Autodesk Fusion 360 part; units mm, degrees
sketch "Skizze1" plane through (0, 0, 0) normal (0, 0, 1) x (1, 0, 0)
  line L0 (0, 0) -> (200, 0)
  line L1 (200, 0) -> (200, 24)
  line L2 (200, 24) -> (0, 24)
  line L3 (0, 24) -> (0, 0)
  line L4 (2, 2) -> (198, 2)
  line L5 (198, 2) -> (198, 22)
  line L6 (198, 22) -> (2, 22)
  line L7 (2, 22) -> (2, 2)
  dimension "d1" = 200
  dimension "d2" = 24
extrude "Extrusion1" add sketch "Skizze1" along normal blind 2 contours L4 L5 L6 L7
extrude "Extrusion2" add sketch "Skizze1" along normal blind 124
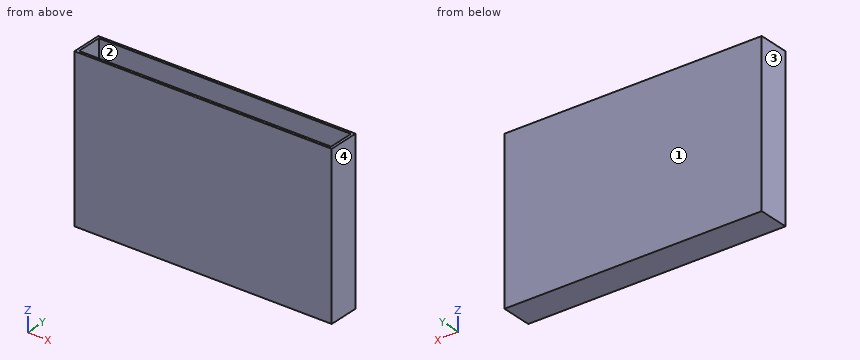
The model under review builds one solid part; all positions refer to its coordinate system, in mm. Face numbers are marked on the shaded views. Give positions to 0.01 mm unless a question says otherwise; leave off trailing zeros. Order: outer loops, then holes, each group sorted by start corner. A loop starts at its lowest first (then second) coordinate and runs counter-clockwise, first axis right, second up. Notation, with made-up numbers: (13.25, 74) -> (50.25, 74) arc R16 cw to (50.25, 86) -> close; hole circle Ø4 at (32.25, 14). An arc over 180 degrees is marked (long way). Write item = value, one per line. Start each with the question number.
(1) Take a section at B-B (x = 76). Write out the cut boundary in (y, z).
(2) Draft analysis for pull direction X (two halves, no side actions). For the marked faces 1, 2, 3 and 4, state which applies: +X half, -X half, draft (parallel to the pull), parting line (faces both ways), or undercut.
(3) Take a section at A-A (z = 58). Write out the cut boundary in (x, y).
(4) Take a section at C-C (y = 5.25). Write out the cut boundary in (x, z), plus the area to 3 significant figures.
(5) For L1, parallel to X at y = 7, z = 83; L2, parallel to Y at x = 178.5, z = 23.5; L3, parallel to Z at x = 105, y = 10, list the stretches that pass through material, from the lowest coordinate up. Write a range as from..to.
Returned:
q1.outline = (0, 0) -> (24, 0) -> (24, 124) -> (22, 124) -> (22, 2) -> (2, 2) -> (2, 124) -> (0, 124) -> close
q2.face_1 = draft
q2.face_2 = undercut
q2.face_3 = -X half
q2.face_4 = +X half
q3.outline = (0, 0) -> (200, 0) -> (200, 24) -> (0, 24) -> close; hole (2, 2) -> (198, 2) -> (198, 22) -> (2, 22) -> close
q4.outline = (0, 0) -> (200, 0) -> (200, 124) -> (198, 124) -> (198, 2) -> (2, 2) -> (2, 124) -> (0, 124) -> close
q4.area = 888 mm²
q5.L1 = 0..2, 198..200
q5.L2 = 0..2, 22..24
q5.L3 = 0..2
